Source: three-view drawing plus pictorial views. Frame: mm from the lowest corner of the part. Coordinates: 2 decimals unless noted, no trailing zeros. Loops run counter-clockwise (first coordinate to the right, second up) from the corner with the lowest first, then second, coordinate; pieces in that order, holes last. Notation, with made-up numbers: M 34,36.5 L 91,36.5 A26 cw 91,67.5 Z; hole C 14.5,77 d9. An arc over 180 degrees is marked long. Write each question's results on one line, items separated by ' | '. Start each with the question number.
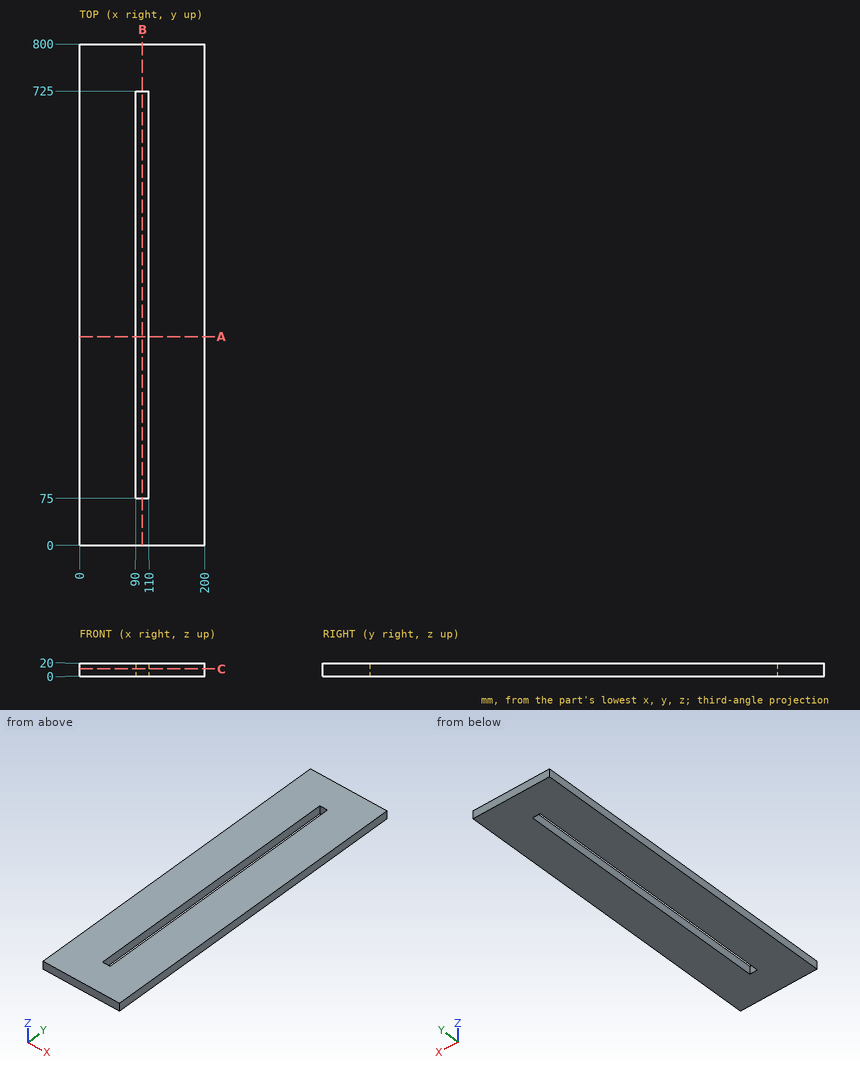
Item 1: Section A-A, the plane y = 333. Return loops of the section in (x, z).
Item 2: Ray query, L1, parallel to X at y = 685.5, z = 5.5; L2, parallel to Y at x = 95, z = 8.25. Return the intervals inside material, ascending. Write a range as [from, to].
Item 3: Section C-C, the plane z = 11.25. Return loops of the section in (x, y).
Item 4: Section B-B, the plane x = 100. Return loops of the section in (y, z).
Solutions:
1) outline: M 0,0 L 90,0 L 90,20 L 0,20 Z; M 110,0 L 200,0 L 200,20 L 110,20 Z
2) L1: x = [0, 90], [110, 200] | L2: y = [0, 75], [725, 800]
3) outline: M 0,0 L 200,0 L 200,800 L 0,800 Z; hole M 90,75 L 110,75 L 110,725 L 90,725 Z
4) outline: M 0,0 L 75,0 L 75,20 L 0,20 Z; M 725,0 L 800,0 L 800,20 L 725,20 Z
